from build123d import *

# Parameters (mm, degrees)
HEADCHAMFER_SIZE   = 1.5
CUT_EXTRUDE1_DEPTH = 2.3
CUT_EXTRUDE2_DEPTH = 2.8
BODYCHAMFER_SIZE   = 0.75


with BuildPart() as part:
    # Sketch2 → Base (revolve)
    with BuildSketch(Plane.XY, mode=Mode.PRIVATE) as base_sk:
        with BuildLine():
            Line((0, 0), (0, 9))
            Line((0, 9), (6.4, 9))
            Line((6.4, 9), (6.4, 6.8))
            ThreePointArc((6.4, 6.8), (6.634314575, 6.234314575), (7.2, 6))
            Line((7.2, 6), (56.4, 6))
            Line((56.4, 6), (56.4, 0))
            Line((56.4, 0), (0, 0))
        make_face()
    revolve(base_sk.sketch.rotate(Axis((-56.067516779, 0, 0), (1, 0, 0)), 90), axis=Axis((-56.067516779, 0, 0), (1, 0, 0)))

    # HeadChamfer
    headchamfer_edges = [part.edges().sort_by_distance(p)[0] for p in [
        (0, 0, -9),
    ]]
    chamfer(headchamfer_edges, length=HEADCHAMFER_SIZE)

    # Sketch3 → Cut-Extrude1 (cut)
    with BuildSketch(Plane.XY.offset(6)):
        with BuildLine():
            Line((24.4, 1.5), (34.4, 1.5))
            ThreePointArc((34.4, 1.5), (35.9, 0), (34.4, -1.5))
            Line((34.4, -1.5), (24.4, -1.5))
            ThreePointArc((24.4, -1.5), (22.9, 0), (24.4, 1.5))
        make_face()
    extrude(amount=-CUT_EXTRUDE1_DEPTH, mode=Mode.SUBTRACT)

    # Sketch4 → Cut-Extrude2 (cut)
    with BuildSketch(Plane.XY.offset(6)):
        with BuildLine():
            Line((24.4, 1.5), (28.4, 1.5))
            ThreePointArc((28.4, 1.5), (29.9, 0), (28.4, -1.5))
            Line((28.4, -1.5), (24.4, -1.5))
            ThreePointArc((24.4, -1.5), (22.9, 0), (24.4, 1.5))
        make_face()
    extrude(amount=-CUT_EXTRUDE2_DEPTH, mode=Mode.SUBTRACT)

    # BodyChamfer
    bodychamfer_edges = [part.edges().sort_by_distance(p)[0] for p in [
        (56.4, 0, -6),
    ]]
    chamfer(bodychamfer_edges, length=BODYCHAMFER_SIZE)


solid = part.part
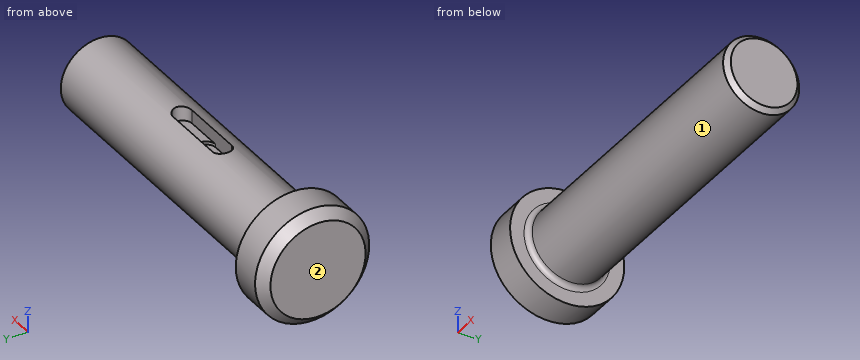
Can you work these out from the model? Positions are in its coordinate system, mm. Face numbers are marked on the shaded views. A direction names the side the tool comes from. Coordinates: 2 decimals unless noted, no trailing zeros. Order: outer loops, then holes, each group sorted by start corner. A loop starts at its lowest first (then second) coordinate and runs counter-clockwise, first axis right, second up. Notation, with made-up numbers: M -20,-38 L -2,-38 A7 cw -2,-34 Z; hole C 30.25,89.25 d6. An arc over 180 degrees is marked long. Write item = value, one per line.
(1) For the marked faces 1 and 2, which set-ups out of +Z, -Z, +X, -X, +Y, -Y let a thin tool reach every point of the face, with its end or its side?
Results are:
face_1 = +X
face_2 = +Z, -Z, -X, +Y, -Y
(2) Suppose I cut it at A-A on z = 0. Please give me the cut outline in (x, y).
Results are:
outline = M 0,-7.5 L 1.5,-9 L 6.4,-9 L 6.4,-6.8 A0.8 cw 7.2,-6 L 55.65,-6 L 56.4,-5.25 L 56.4,5.25 L 55.65,6 L 7.2,6 A0.8 cw 6.4,6.8 L 6.4,9 L 1.5,9 L 0,7.5 Z
(3) Suppose I cut it at C-C on x = 40.5. Please give me the cut outline in (y, z).
Results are:
outline = C 0,0 d12
(4) Suppose I cut it at D-D on x = 4.5. Please give me the cut outline in (y, z), plus the area to 3 significant figures.
Results are:
outline = C 0,0 d18
area = 254 mm2
(5) I need wall thicknesses on line 1 along X through (y, z) = (-5.25, 4.75); line 2 along Z through (x, y) = (4, -0.25); line 3 along X through (y, z) = (-1, 3.75). Which ranges of each line are inside material? Lowest first, please. Write a range as [from, to].
Results are:
line_1 = [0, 6.4]
line_2 = [-9, 9]
line_3 = [0, 23.28], [35.52, 56.4]
(6) For pin 1 Ø5 at (x, y) = (48, 3) entering from +Z; pin 2 Ø4 at (y, z) = (3.5, -5.5) entering from -X; pin 3 Ø6 at (x, y) = (41, 5.5) entering from -Z; pin 4 Ø1.3 at (x, z) = (30, 4.5) entering from +Y, each with a flat end and sliding along its axis, tell me the tip position at first contact or that it passes through.
Results are:
pin_1 = 5.98
pin_2 = 0
pin_3 = -5.45
pin_4 = 4.6
(7) Suppose I cut it at B-B on y = 0. Please give me the cut outline in (x, z).
Results are:
outline = M 0,-7.5 L 1.5,-9 L 6.4,-9 L 6.4,-6.8 A0.8 cw 7.2,-6 L 55.65,-6 L 56.4,-5.25 L 56.4,5.25 L 55.65,6 L 35.9,6 L 35.9,3.7 L 29.9,3.7 L 29.9,3.2 L 22.9,3.2 L 22.9,6 L 7.2,6 A0.8 cw 6.4,6.8 L 6.4,9 L 1.5,9 L 0,7.5 Z
